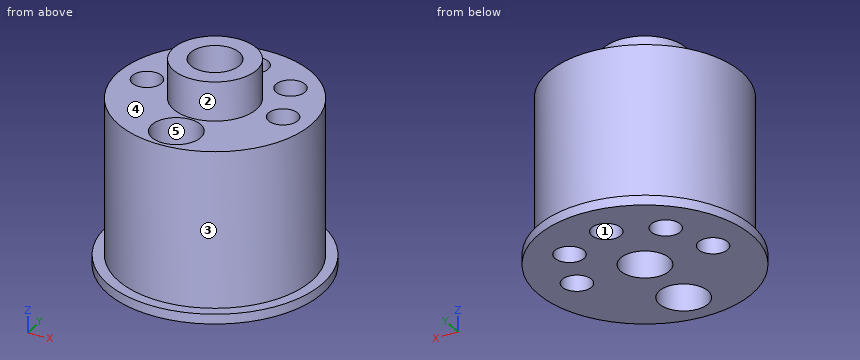
```python
from build123d import *

# Parameters (mm, degrees)
F0_R     = 4.25
F0_R_2   = 2.5
F1_DEPTH = 21
F0_R_3   = 9.9
F0_R_4   = 1.5
F2_DEPTH = 17
F0_R_5   = 11
F3_DEPTH = 1


with BuildPart() as f1:
    # F0 (on Top) → F1 (new body)
    with BuildSketch(Plane.XY):
        Circle(F0_R)
        Circle(F0_R_2, mode=Mode.SUBTRACT)
    extrude(amount=F1_DEPTH)

    # F0 (on Top) → F2 (join)
    with BuildSketch(Plane.XY):
        Circle(F0_R_3)
        with Locations((0, -7)):
            Circle(F0_R_2, mode=Mode.SUBTRACT)
        with Locations((-7, 0)):
            Circle(F0_R_4, mode=Mode.SUBTRACT)
        with Locations((-4.95, 4.949495)):
            Circle(F0_R_4, mode=Mode.SUBTRACT)
        Circle(F0_R, mode=Mode.SUBTRACT)
        with Locations((4.95, 4.949495)):
            Circle(F0_R_4, mode=Mode.SUBTRACT)
        with Locations((7, 0)):
            Circle(F0_R_4, mode=Mode.SUBTRACT)
        with Locations((0, 7)):
            Circle(F0_R_4, mode=Mode.SUBTRACT)
    extrude(amount=F2_DEPTH)

    # F0 (on Top) → F3 (join)
    with BuildSketch(Plane.XY):
        Circle(F0_R_5)
        Circle(F0_R_3, mode=Mode.SUBTRACT)
    extrude(amount=F3_DEPTH)


solid = f1.part
```
Verification items for the finished model (mm, model axes). Face numbers are marked on the shaded views. A direction names the side the tool comes from. Coordinates: 2 decimals unless noted, no trailing zeros. Write each loop counter-clockwise with the first axis right and the second up, starting at its lowest first coordinate (ties: lowest second). Pieces come first, ordered by that corner, then holes. Notation, with made-up numbers: M -17.75,-34 L -4.75,-34 A35 ccw -4.75,5 Z; hole C 31.25,24 d11. An arc over 180 degrees is marked long. One line per item, written item: value.
Item 1: Access from +Z, -Z, +X, -X, +Y, -Y to the whole of each face (thin tool, end or side, straight path). Record for the marked faces 1 and 2.
Check sheet entries:
face 1: +Z, -Z
face 2: +Z
Item 2: Section check D-D, the plane x = -4.95. Record the boundary of the cut face in (y, z), plus the area to 3 significant figures.
Check sheet entries:
outline: M -9.82,0 L 3.45,0 L 3.45,17 L -8.57,17 L -8.57,1 L -9.82,1 Z; M 6.45,0 L 9.82,0 L 9.82,1 L 8.57,1 L 8.57,17 L 6.45,17 Z
area: 243 mm^2
Item 3: Mould release check, pull along Y, two halves, no side actions. Record for the marked faces 3, 4 and 5: pulls with the +Y half, pulls with the -Y half, needs draft (parallel to the pull), parting line crosses it, or undercut.
Check sheet entries:
face 3: parting line crosses it
face 4: needs draft
face 5: undercut
Item 4: Section check B-B, the plane y = 0. Record the boundary of the cut face in (x, z).
Check sheet entries:
outline: M -11,0 L -8.5,0 L -8.5,17 L -9.9,17 L -9.9,1 L -11,1 Z; M -5.5,0 L -2.5,0 L -2.5,21 L -4.25,21 L -4.25,17 L -5.5,17 Z; M 2.5,0 L 5.5,0 L 5.5,17 L 4.25,17 L 4.25,21 L 2.5,21 Z; M 8.5,0 L 11,0 L 11,1 L 9.9,1 L 9.9,17 L 8.5,17 Z
Item 5: Gauge pin test, flat ends, axial feed: pin 1 Ø1.5 at (x, z) = (1, 11.5) entering from -Y; pin 2 Ø2.5 at (x, y) = (-4.95, 4.95) entering from +Z; pin 3 Ø10 at (x, z) = (5.5, 3.5) entering from -Y; pin 4 Ø8 at (y, z) = (4.5, 18.5) entering from -X. Record the tip position at first contact, or that the pin passes through.
Check sheet entries:
pin 1: stops at y = -9.9
pin 2: passes through
pin 3: stops at y = -10.94
pin 4: stops at x = -9.87
Item 6: Scan lines: line 1 along Y through (x, z) = (0, 9.25); line 2 along Y through (x, z) = (-2.25, 16); line 3 along Z through (x, y) = (-4, 3). Record each from-to range of solid material in increasing order.
Check sheet entries:
line 1: y = -9.9 to -9.5, -4.5 to -2.5, 2.5 to 5.5, 8.5 to 9.9
line 2: y = -9.64 to -8.09, -5.91 to -1.09, 1.09 to 9.64
line 3: z = 0 to 17
Item 7: Section check C-C, the plane y = 3.75. Record the boundary of the cut face in (x, z), plus the area to 3 significant figures.
Check sheet entries:
outline: M -10.34,0 L -5.85,0 L -5.85,17 L -9.16,17 L -9.16,1 L -10.34,1 Z; M -4.05,0 L 4.05,0 L 4.05,17 L 2,17 L 2,21 L -2,21 L -2,17 L -4.05,17 Z; M 5.85,0 L 10.34,0 L 10.34,1 L 9.16,1 L 9.16,17 L 5.85,17 Z
area: 269 mm^2
Item 8: Section check A-A, the plane x = 0. Record the boundary of the cut face in (y, z), plus the area to 3 significant figures.
Check sheet entries:
outline: M -11,0 L -9.5,0 L -9.5,17 L -9.9,17 L -9.9,1 L -11,1 Z; M -4.5,0 L -2.5,0 L -2.5,21 L -4.25,21 L -4.25,17 L -4.5,17 Z; M 2.5,0 L 5.5,0 L 5.5,17 L 4.25,17 L 4.25,21 L 2.5,21 Z; M 8.5,0 L 11,0 L 11,1 L 9.9,1 L 9.9,17 L 8.5,17 Z
area: 132 mm^2
